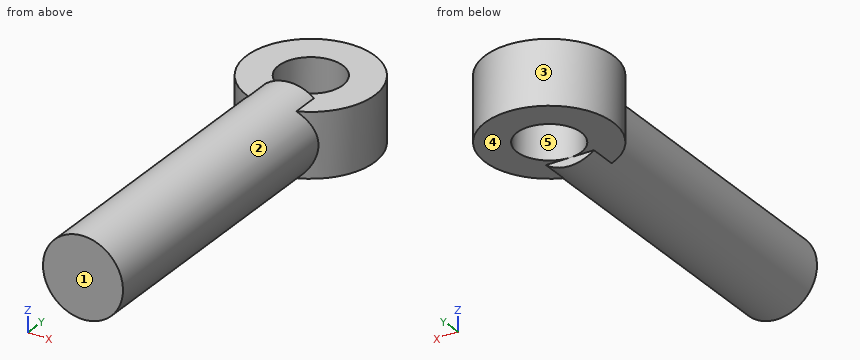
from build123d import *

# Parameters (mm, degrees)
SKETCH1_R      = 1.5875
EXTRUDE1_DEPTH = 12.7
SKETCH2_R      = 2.54
SKETCH2_R_2    = 1.27
EXTRUDE2_DEPTH = 1.27


with BuildPart() as part:
    # Sketch1 → Extrude1 (new body)
    with BuildSketch(Plane(origin=(0, 0, 0), x_dir=(1, 0, 0), z_dir=(0, 1, 0))):
        with Locations(Location((0, 0, 0), (0, 0, 270))):
            Circle(SKETCH1_R)
    extrude(amount=EXTRUDE1_DEPTH)

    # Sketch2 → Extrude2 (add, symmetric)
    with BuildSketch(Plane.XY):
        with Locations((0, 13.97)):
            Circle(SKETCH2_R)
        with Locations(Location((0, 13.97, 0), (0, 0, 270))):
            Circle(SKETCH2_R_2, mode=Mode.SUBTRACT)
    extrude(amount=EXTRUDE2_DEPTH, both=True)


solid = part.part
Source: CAD feature listing. Evaluate the final solid. Frame: model axes, mm. Face numbers are marked on the shaded views. A direction names the side the tool comes from. Coordinates: 2 decimals unless noted, no trailing zeros. Order: outer loops, then holes, each group sorted by start corner. A loop starts at its lowest first (then second) coordinate and runs counter-clockwise, first axis right, second up. Notation, with made-up numbers: M 73,23 L 92,23 A31 ccw 92,60 Z; hole C 27.25,32 d5. An arc over 180 degrees is marked long. Write each question's results on one line, items separated by ' | '. Start each with the question number.
1. Section A-A, the plane y = 13.97. Return the cut outline in (x, z), then the cut area to 3 significant figures.
2. Draft query along Y for the marked faces 3, 4 and 5. Return one class per face: +Y half, -Y half, draft (parallel to the pull), parting line (faces both ways), or undercut.
3. Section B-B, the plane x = -0.45. Return the cut outline in (y, z), then the cut area to 3 significant figures.
4. Reachability of the marked faces 1 and 2 from +Z, -Z, +X, -X, +Y, -Y: full face, straight path, thin tool, end or side. Return the list, or none.
5. Material intervals for L1, parallel to X at y = 13.97, z = 0.3; L2, parallel to X at y = 4.5, z = 0.1; L3, parallel to Y at x = -0.7, z = 0.8, sorted ascending.
6. Pin query (flat end, axial travel): pin 1 (3 mm diameter, centred on x = 0, y = 13.97, fed in from +Z); pin 2 (1 mm diameter, centred on y = 10, z = -1, fed in from -X). Return the tip coordinate at first contact, or that it passes through.
7. Section D-D, the plane y = 5. Return the cut outline in (x, z) (1 decimal).
8. Section C-C, the plane z = 0. Return the cut outline in (x, y), then the cut area to 3 significant figures.
Solution:
1) outline: M -2.54,-1.27 L -1.27,-1.27 L -1.27,1.27 L -2.54,1.27 Z; M 1.27,-1.27 L 2.54,-1.27 L 2.54,1.27 L 1.27,1.27 Z | area: 6.45 mm²
2) face 3: parting line | face 4: draft | face 5: undercut
3) outline: M 0,-1.52 L 12.7,-1.52 L 12.7,-1.27 L 12.78,-1.27 L 12.78,1.27 L 12.7,1.27 L 12.7,1.52 L 0,1.52 Z; M 15.16,-1.27 L 16.47,-1.27 L 16.47,1.27 L 15.16,1.27 Z | area: 42.2 mm²
4) face 1: +Z, -Z, +X, -X, -Y | face 2: -Y
5) L1: -2.54 to -1.27, 1.27 to 2.54 | L2: -1.58 to 1.58 | L3: 0 to 12.91, 15.03 to 16.41
6) pin 1: z = 1.59 | pin 2: x = -1.51
7) outline: C 0,0 d3.2
8) outline: M -1.59,0 L 1.59,0 L 1.59,11.99 A2.54 ccw long -1.59,11.99 Z; hole C 0,13.97 d2.54 | area: 52.1 mm²
